Here's how the part is built. I have some questions about the finished solid (model axes, mm). Face numbers are marked on the shaded views. A direction names the side the tool comes from. Round coordinates to 2 decimals unless told otherwise and drop trailing zeros. Write each loop counter-clockwise with the first axis right and the second up, starting at its lowest first coordinate (ties: lowest second). Pieces come first, ordered by that corner, then holes. Notation, with made-up numbers: (-16.5, 80.5) -> (1.5, 80.5) arc R21 ccw to (1.5, 110.5) -> close; hole circle Ø5 at (-6, 6.25). An arc over 180 degrees is marked (long way). Put each result on its own line as item: value. Start each with the question number.
1. Which directions (+Z, -Z, +X, -X, +Y, -Y) give clear straight access to the entire face, cutting with the end or side of a thin tool? Please do the marked faces 1, 2 and 3.
2. For pin 1 (1.5 mm diameter, centred on x = 114, y = 53.5, fed in from +Z); pin 2 (10 mm diameter, centred on x = 167, y = 11, fed in from +Z); pin 3 (10 mm diameter, centred on x = 174.5, y = 79, fed in from +Z), each with a flat end and sliding along its axis, tell me the tip position at first contact or that it passes through.
3. Suppose I cut it at D-D (x = 22). Please give me the cut outline in (y, z).
4. Suppose I cut it at C-C (y = 10). Please give me the cut outline in (x, z), then the cut area to 3 significant figures.
5. Suppose I cut it at B-B (x = 170). Please give me the cut outline in (y, z).
6. Suppose I cut it at A-A (z = 183). Please give me the cut outline in (x, y).
7. I need wall thicknesses on probe 1 along Z at (x, y) = (170, 19.5); probe 2 along X at (y, z) = (30, 183); probe 3 along Z at (x, y) = (170, 27.75). Which ranges of each line are inside material? Lowest first, please. Write a range as from..to.
8. We'd pull the mould along Y, two halves only. Please class the marked faces 4, 5, 6 and 7: +Y half, -Y half, draft (parallel to the pull), parting line (faces both ways), or undercut.
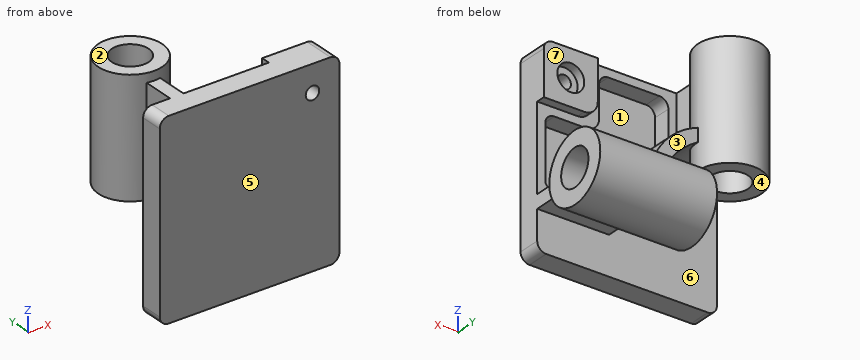
```python
from build123d import *

# Parameters (mm, degrees)
SKETCH1_W                               = 200
SKETCH1_H                               = 213
BOSS_EXTRUDE1_DEPTH                     = 25
SKETCH2_W                               = 60
SKETCH2_H                               = 60
BOSS_EXTRUDE2_DEPTH                     = 10
CUT_EXTRUDE1_DEPTH                      = 20
BOSS_EXTRUDE3_DEPTH                     = 70
BOSS_EXTRUDE5_DEPTH                     = 10
BOSS_EXTRUDE5_DEPTH_BACK                = 120
SKETCH6_R                               = 35.5
BOSS_EXTRUDE6_DEPTH                     = 10
BOSS_EXTRUDE6_DEPTH_BACK                = 120
SKETCH7_R                               = 38.333333333
F_12_0_41_DIAMETER_HOLE1_D              = 41
F_12_0MM_DOWEL_HOLE1_D                  = 41
CBORE_FOR_M8_HEX_HEAD_BOLT1_D           = 15
CBORE_FOR_M8_HEX_HEAD_BOLT1_CBORE_D     = 30
CBORE_FOR_M8_HEX_HEAD_BOLT1_CBORE_DEPTH = 10
FILLET1_R                               = 10
FILLET2_R                               = 15


with BuildPart() as part:
    # Sketch1 → Boss-Extrude1 (new body)
    with BuildSketch(Plane(origin=(0, 0, 0), x_dir=(1, 0, 0), z_dir=(0, 1, 0))):
        with Locations((100, -106.5)):
            Rectangle(SKETCH1_W, SKETCH1_H)
    extrude(amount=BOSS_EXTRUDE1_DEPTH)

    # Sketch2 → Boss-Extrude2 (add)
    with BuildSketch(Plane(origin=(0, 25, 0), x_dir=(1, 0, 0), z_dir=(0, 1, 0))):
        with Locations((170, -183)):
            Rectangle(SKETCH2_W, SKETCH2_H)
    extrude(amount=BOSS_EXTRUDE2_DEPTH)

    # Sketch5 → Cut-Extrude1 (cut)
    with BuildSketch(Plane(origin=(0, 25, 0), x_dir=(1, 0, 0), z_dir=(0, 1, 0))):
        with BuildLine():
            Line((191, -73.400231973), (191, -134))
            ThreePointArc((191, -134), (188.071067812, -141.071067812), (181, -144))
            Line((181, -144), (145.524792721, -144))
            ThreePointArc((145.524792721, -144), (135.254213293, -148.254213293), (131, -158.524792721))
            Line((131, -158.524792721), (131, -194))
            ThreePointArc((131, -194), (128.071067812, -201.071067812), (121, -204))
            Line((121, -204), (64, -204))
            ThreePointArc((64, -204), (56.928932188, -201.071067812), (54, -194))
            Line((54, -194), (54, -155.925475005))
            ThreePointArc((54, -155.925475005), (56.596304606, -149.203474223), (63.037058903, -145.97194576))
            ThreePointArc((63.037058903, -145.97194576), (110.669303842, -123.548265985), (133.270417334, -75.999955378))
            ThreePointArc((133.270417334, -75.999955378), (136.512099917, -69.583786471), (143.22028722, -67))
            Line((143.22028722, -67), (181.67038746, -67))
            ThreePointArc((181.67038746, -67), (187.327344227, -68.753859076), (191, -73.400231973))
        make_face()
    extrude(amount=-CUT_EXTRUDE1_DEPTH, mode=Mode.SUBTRACT)

    # Sketch3 → Boss-Extrude3 (add)
    with BuildSketch(Plane(origin=(0, 25, 0), x_dir=(1, 0, 0), z_dir=(0, 1, 0))):
        with BuildLine():
            Line((30, -213), (30, -133))
            ThreePointArc((30, -133), (93.639610307, -106.639610307), (120, -43))
            Line((120, -43), (200, -43))
            Line((200, -43), (200, -58))
            Line((200, -58), (128.786796564, -58))
            ThreePointArc((128.786796564, -58), (104.246212025, -117.246212025), (45, -141.786796564))
            Line((45, -141.786796564), (45, -213))
            Line((45, -213), (30, -213))
        make_face()
    extrude(amount=BOSS_EXTRUDE3_DEPTH)

    # Sketch6 → Boss-Extrude5 (add, two sides: drawn at the far end of the back side and taken through both)
    with BuildSketch(Plane.XY.offset(213).offset(-BOSS_EXTRUDE5_DEPTH_BACK)):
        with Locations((37.5, 95)):
            Circle(SKETCH6_R)
    extrude(amount=BOSS_EXTRUDE5_DEPTH + BOSS_EXTRUDE5_DEPTH_BACK)

    # Sketch7 → Boss-Extrude6 (add, two sides: drawn at the far end of the back side and taken through both)
    with BuildSketch(Plane(origin=(200, 0, 0), x_dir=(0, 0, -1), z_dir=(1, 0, 0)).offset(-BOSS_EXTRUDE6_DEPTH_BACK)):
        with Locations((-50.5, 95)):
            Circle(SKETCH7_R)
    extrude(amount=BOSS_EXTRUDE6_DEPTH + BOSS_EXTRUDE6_DEPTH_BACK)

    # Ø12.0 (41) Diameter Hole1 (through all)
    with Locations(Plane(origin=(210, 0, 0), x_dir=(0, 0, -1), z_dir=(1, 0, 0))):
        with Locations((-50.5, 95)):
            Hole(F_12_0_41_DIAMETER_HOLE1_D / 2)

    # Ø12.0mm Dowel Hole1 (through all)
    with Locations(Plane.XY.offset(223)):
        with Locations((37.5, 95)):
            Hole(F_12_0MM_DOWEL_HOLE1_D / 2)

    # CBORE for M8 Hex Head Bolt1 (through all)
    with Locations(Plane(origin=(0, 35, 0), x_dir=(1, 0, 0), z_dir=(0, 1, 0))):
        with Locations((170, -183)):
            CounterBoreHole(CBORE_FOR_M8_HEX_HEAD_BOLT1_D / 2, CBORE_FOR_M8_HEX_HEAD_BOLT1_CBORE_D / 2, CBORE_FOR_M8_HEX_HEAD_BOLT1_CBORE_DEPTH)

    # Fillet1
    fillet1_edges = [part.edges().sort_by_distance(p)[0] for p in [
        (0, 12.5, 0),
        (200, 12.5, 0),
        (200, 17.5, 213),
        (0, 12.5, 213),
    ]]
    fillet(fillet1_edges, radius=FILLET1_R)

    # Fillet2
    fillet2_edges = [part.edges().sort_by_distance(p)[0] for p in [
        (140, 30, 153),
    ]]
    fillet(fillet2_edges, radius=FILLET2_R)


solid = part.part
```
Verdict:
1. face 1: none
1. face 2: +Z, +X, -X, +Y, -Y
1. face 3: +Z, +X, +Y
2. pin 1: stops at z = 106.6
2. pin 2: stops at z = 213
2. pin 3: stops at z = 87.22
3. outline: (0, 0) -> (25, 0) -> (25, 213) -> (0, 213) -> close; (63.06, 93) -> (81.58, 93) -> (81.58, 223) -> (63.06, 223) -> close; (108.42, 93) -> (126.94, 93) -> (126.94, 223) -> (108.42, 223) -> close
4. outline: (0, 10) arc R10 ccw to (10, 0) -> (190, 0) arc R10 ccw to (200, 10) -> (200, 203) arc R10 ccw to (190, 213) -> (10, 213) arc R10 ccw to (0, 203) -> close; hole (54, 155.93) arc R10 ccw to (63.04, 145.97) arc R78.15 cw to (133.27, 76) arc R10 ccw to (143.22, 67) -> (181.67, 67) arc R10 ccw to (191, 73.4) -> (191, 134) arc R10 ccw to (181, 144) -> (145.52, 144) arc R14.52 cw to (131, 158.52) -> (131, 194) arc R10 ccw to (121, 204) -> (64, 204) arc R10 ccw to (54, 194) -> close; hole circle Ø15 at (170, 183)
4. area: 32,300 mm^2
5. outline: (0, 0) -> (25, 0) -> (25, 43) -> (57.41, 43) arc R38.33 ccw (long way) to (57.41, 58) -> (25, 58) -> (25, 67) -> (5, 67) -> (5, 144) -> (25, 144) -> (25, 153) -> (35, 153) -> (35, 168) -> (25, 168) -> (25, 175.5) -> (0, 175.5) -> close; (0, 190.5) -> (25, 190.5) -> (25, 198) -> (35, 198) -> (35, 213) -> (0, 213) -> close; hole circle Ø41 at (95, 50.5)
6. outline: (0, 0) -> (162.5, 0) -> (162.5, 25) -> (155, 25) -> (155, 35) -> (140, 35) -> (140, 25) -> (131, 25) -> (131, 5) -> (54, 5) -> (54, 25) -> (45, 25) -> (45, 60.3) arc R35.5 ccw (long way) to (30, 60.3) -> (30, 25) -> (0, 25) -> close; (177.5, 0) -> (200, 0) -> (200, 35) -> (185, 35) -> (185, 25) -> (177.5, 25) -> close; hole circle Ø41 at (37.5, 95)
7. probe 1: z = 0..67, 144..175.5, 190.5..213
7. probe 2: x = 30..45, 140..155, 185..200
7. probe 3: z = 43..58, 153..168, 198..213
8. face 4: draft
8. face 5: -Y half
8. face 6: undercut
8. face 7: +Y half
